Part model, mm, in its own coordinate system. A direction names the side the tool comes from. Round coordinates to 2 decimals unless told otherwise and drop trailing zeros. Order: outer loops, then holes, each group sorted by start corner. A loop starts at its lowest first (then second) coordinate and runs counter-clockwise, first axis right, second up. Notation, with made-up numbers: (28, 73.5) -> (66, 73.5) arc R35 ccw to (66, 109.5) -> close; hole circle Ø7 at (5.25, 7). An arc over 180 degrees is marked (long way). Answer as a JSON object with one key per item and string values. Group by question number.
```python
from build123d import *

# Parameters (mm, degrees)
SKETCH_R      = 50
SKETCH_R_2    = 7.5
SKETCH_R_3    = 10
PAD_DEPTH     = 5
SKETCH001_R   = 17.5
SKETCH001_R_2 = 10
PAD001_DEPTH  = 15
SKETCH002_R   = 45
POCKET_DEPTH  = 3
FILLET_R      = 2


with BuildPart() as part:
    # Sketch (on XY_Plane of Origin) → Pad (new body)
    with BuildSketch(Plane.XY):
        Circle(SKETCH_R)
        with Locations((0, 29.995833)):
            Circle(SKETCH_R_2, mode=Mode.SUBTRACT)
        with Locations((-29.5, 0)):
            Circle(SKETCH_R_2, mode=Mode.SUBTRACT)
        with Locations((30.5, 0)):
            Circle(SKETCH_R_2, mode=Mode.SUBTRACT)
        with Locations((0, -29.995833)):
            Circle(SKETCH_R_2, mode=Mode.SUBTRACT)
        Circle(SKETCH_R_3, mode=Mode.SUBTRACT)
    extrude(amount=PAD_DEPTH)

    # Sketch001 (on Face8 of Pad) → Pad001 (join)
    with BuildSketch(Plane.XY.offset(5)):
        Circle(SKETCH001_R)
        Circle(SKETCH001_R_2, mode=Mode.SUBTRACT)
    extrude(amount=PAD001_DEPTH)

    # Sketch002 (on Face2 of Pad001) → Pocket (cut)
    with BuildSketch(Plane(origin=(0, 0, 0), x_dir=(1, 0, 0), z_dir=(0, 0, -1))):
        Circle(SKETCH002_R)
    extrude(amount=-POCKET_DEPTH, mode=Mode.SUBTRACT)

    # Fillet
    fillet_edges = [part.edges().sort_by_distance(p)[0] for p in [
        (-17.5, 0, 20),
        (-17.5, 0, 5),
        (-50, 0, 5),
        (-50, 0, 0),
    ]]
    fillet(fillet_edges, radius=FILLET_R)


solid = part.part
```
Q1. Two-plate mould, pull along Y, no slides. Class faces 4 (the cylindrical face through (-0.98, 37.43, 3.99)), 5 (the cylindrical face through (-13.887, -10.648, 12.423)), 6 (the flat face through (3, -10, 20)), 7 (the flat face through (-1, -11, 3)): +Y half, -Y half, draft (parallel to the pull), parting line (faces both ways), or undercut.
Q2. Band-saw the part on B-B (z = 16). List the corners of the cut face in (x, y), plus the area to 3 significant figures.
Q3. Wall check: line 1 (Y direction, x = 0, z = 2.15); line 2 (Y direction, x = 0, z = 3.85); line 3 (Z direction, x = 23, y = -10). Give the ranges that are in metal, low to high. Write a range as [from, to].
Q4. Band-saw the part on A-A (y = 0). Count the separate pieces of the cut face and the enclosed holes in it, plus the area to 3 significant figures.
Q5. Drop flat-ended pins along their axis: pin 1 Ø8 at (y, z) = (-9, 12.5) entering from +X; pin 2 Ø6 at (x, z) = (6.5, 14) entering from -Y; pin 3 Ø12 at (x, y) = (0, 0) entering from +Z; pin 4 Ø19.5 at (x, y) = (30.5, 0) entering from +Z. Give the stop position or say it passes through.
Q6. Which spindle directions (+Z, -Z, +X, -X, +Y, -Y) get a long thin tool onto all of the face, cutting with end or side? Do faces 1 (the cylindrical face through (-37, 0, 4)), 2 (the cylindrical face through (20.765, 39.923, 1.479)), 3 (the flat face through (21, 1, 5)). Say none if no direction does.
Completed:
{
 "1": {"face 4": "undercut", "face 5": "parting line", "face 6": "draft", "face 7": "undercut"},
 "2": {"outline": "circle Ø35 at (0, 0); hole circle Ø20 at (0, 0)", "area": "648 mm2"},
 "3": {"line 1": "[-50, -45], [45, 50]", "line 2": "[-49.81, -37.5], [-22.5, -10], [10, 22.5], [37.5, 49.81]", "line 3": "[3, 5]"},
 "4": {"separate pieces": "4", "enclosed holes": "0", "area": "352 mm2"},
 "5": {"pin 1": "x = 16.77", "pin 2": "y = -17.15", "pin 3": "through", "pin 4": "z = 5"},
 "6": {"face 1": "+Z, -Z", "face 2": "-Z", "face 3": "+Z"}
}
